The listing builds one solid part. Answer for the finished solid, in the listing's coordinates (mm). A direction names the side the tool comes from. Give positions to 0.01 mm unless a question says otherwise; leave off trailing zeros. Loops run counter-clockwise (first coordinate to the right, second up) from the corner with the lowest first, then second, coordinate; pieces in that order, holes last. Notation, with made-up numbers: (-7, 60) - (50, 60) arc R22 cw to (50, 72) - close; hole circle Ø5 at (42, 78.5). An arc over 180 degrees is marked (long way). Answer as CSV lines item,"result". Start each with the question number.
1) For faces 1 (the face through (2.311, 19.581, -10.407)), 2 (the face through (16.477, -0.055, 25.844)), 3 (the face through (6, -3.9, -13)), determine the directions among +Z, -Z, +X, -X, +Y, -Y from which every point of the face is accessible in a straight line to the end or side of a thin tool.
2) A cutting plane is placed at B-B (z = 0). Determine the outline of the cut face in (x, y) (3 decimals).
3) Flat-ended cylindrical pins translate along their axes: pin 1 (15.5 mm diameter, centred on x = 0, z = 0, fed in from +Y); pin 2 (6 mm diameter, centred on x = -16.5, z = -8, fed in from +Y); pin 3 (4 mm diameter, centred on x = -17, y = 1.5, fed in from -Z); pin 4 (8 mm diameter, centred on x = 6.5, y = -10.5, fed in from -Z). Find the tip coordinate at first contact, or state that the pin passes through.
4) A cutting plane is placed at A-A (x = 0). Determine the outline of the cut face in (y, z) (3 decimals), and give its area (3 significant figures).
5) A cutting plane is placed at C-C (y = 7.5). Determine the outline of the cut face in (x, z).
6) Find the intervals of material crossed by line 1 along Z through (x, y) = (0, -5.75); line 2 along Y through (x, z) = (-15, -14.5); line 3 along Z through (x, y) = (0, 18), in increasing order.
7) A cutting plane is placed at D-D (x = 12). Determine the outline of the cut face in (y, z), and give its area (3 significant figures).
```python
from build123d import *

# Parameters (mm, degrees)
F0_R      = 30.65
F0_R_2    = 6
F1_DEPTH  = 3.9
F2_R      = 14.1
F2_R_2    = 6
F3_DEPTH  = 6.4
F4_R      = 9.4
F4_R_2    = 6
F5_DEPTH  = 6.1
F6_R      = 13.9
F7_DEPTH  = 10.2
F8_R      = 12.875
F9_DEPTH  = 0.6
F10_R     = 10.66
F11_DEPTH = 9.9
F12_DEPTH = 24.601


with BuildPart() as f1:
    # F0 (on Front) → F1 (new body, symmetric)
    with BuildSketch(Plane.XZ):
        Circle(F0_R)
        Circle(F0_R_2, mode=Mode.SUBTRACT)
    extrude(amount=F1_DEPTH, both=True)

    # F2 (on face) → F3 (join)
    with BuildSketch(Plane.XZ.offset(3.9)):
        Circle(F2_R)
        Circle(F2_R_2, mode=Mode.SUBTRACT)
    extrude(amount=F3_DEPTH)

    # F4 (on face) → F5 (join)
    with BuildSketch(Plane.XZ.offset(10.3)):
        Circle(F4_R)
        Circle(F4_R_2, mode=Mode.SUBTRACT)
    extrude(amount=F5_DEPTH)

    # F6 (on face) → F7 (join)
    with BuildSketch(Plane(origin=(0, 3.9, 0), x_dir=(-1, 0, 0), z_dir=(0, 1, 0))):
        Circle(F6_R)
    extrude(amount=F7_DEPTH)

    # F8 (on face) → F9 (join)
    with BuildSketch(Plane(origin=(0, 14.1, 0), x_dir=(-1, 0, 0), z_dir=(0, 1, 0))):
        Circle(F8_R)
    extrude(amount=F9_DEPTH)

    # F10 (on face) → F11 (join)
    with BuildSketch(Plane(origin=(0, 14.7, 0), x_dir=(-1, 0, 0), z_dir=(0, 1, 0))):
        Circle(F10_R)
    extrude(amount=F11_DEPTH)

    # F0 (on Front) → F12 (cut, through all)
    with BuildSketch(Plane.XZ):
        Circle(F0_R_2)
    extrude(amount=-F12_DEPTH, mode=Mode.SUBTRACT)


solid = f1.part
```
Ans:
1,face 1,"+Y"
1,face 2,"+Y, -Y"
1,face 3,"-Y"
2,outline,"(-30.65, -3.9) - (-14.1, -3.9) - (-14.1, -10.3) - (-9.4, -10.3) - (-9.4, -16.4) - (-6, -16.4) - (-6, 24.6) - (-10.66, 24.6) - (-10.66, 14.7) - (-12.875, 14.7) - (-12.875, 14.1) - (-13.9, 14.1) - (-13.9, 3.9) - (-30.65, 3.9) - close; (6, -16.4) - (9.4, -16.4) - (9.4, -10.3) - (14.1, -10.3) - (14.1, -3.9) - (30.65, -3.9) - (30.65, 3.9) - (13.9, 3.9) - (13.9, 14.1) - (12.875, 14.1) - (12.875, 14.7) - (10.66, 14.7) - (10.66, 24.6) - (6, 24.6) - close"
3,pin 1,"y = 24.6"
3,pin 2,"y = 3.9"
3,pin 3,"z = -26.73"
3,pin 4,"z = -13.88"
4,outline,"(-16.4, -9.4) - (-10.3, -9.4) - (-10.3, -14.1) - (-3.9, -14.1) - (-3.9, -30.65) - (3.9, -30.65) - (3.9, -13.9) - (14.1, -13.9) - (14.1, -12.875) - (14.7, -12.875) - (14.7, -10.66) - (24.6, -10.66) - (24.6, -6) - (-16.4, -6) - close; (-16.4, 6) - (24.6, 6) - (24.6, 10.66) - (14.7, 10.66) - (14.7, 12.875) - (14.1, 12.875) - (14.1, 13.9) - (3.9, 13.9) - (3.9, 30.65) - (-3.9, 30.65) - (-3.9, 14.1) - (-10.3, 14.1) - (-10.3, 9.4) - (-16.4, 9.4) - close"
4,area,"791 mm2"
5,outline,"circle Ø27.8 at (0, 0); hole circle Ø12 at (0, 0)"
6,line 1,"-14.1 to -6, 6 to 14.1"
6,line 2,"-3.9 to 3.9"
6,line 3,"-10.66 to -6, 6 to 10.66"
7,outline,"(-10.3, -7.4) - (-3.9, -7.4) - (-3.9, -28.2) - (3.9, -28.2) - (3.9, -7.01) - (14.1, -7.01) - (14.1, -4.67) - (14.7, -4.67) - (14.7, 4.67) - (14.1, 4.67) - (14.1, 7.01) - (3.9, 7.01) - (3.9, 28.2) - (-3.9, 28.2) - (-3.9, 7.4) - (-10.3, 7.4) - close"
7,area,"683 mm2"
